```python
from build123d import *

# Parameters (mm, degrees)
SKETCH1_R           = 30.5
SKETCH1_R_2         = 25
BOSS_EXTRUDE1_DEPTH = 1
SKETCH2_R           = 30.5
SKETCH2_R_2         = 29.5
BOSS_EXTRUDE2_DEPTH = 10
SKETCH3_R           = 30.5
SKETCH3_R_2         = 25
BOSS_EXTRUDE3_DEPTH = 1


with BuildPart() as part:
    # Sketch1 → Boss-Extrude1 (new body)
    with BuildSketch(Plane.XY):
        Circle(SKETCH1_R)
        Circle(SKETCH1_R_2, mode=Mode.SUBTRACT)
    extrude(amount=BOSS_EXTRUDE1_DEPTH)

    # Sketch2 → Boss-Extrude2 (add)
    with BuildSketch(Plane(origin=(0, 0, 0), x_dir=(-1, 0, 0), z_dir=(0, 0, -1))):
        Circle(SKETCH2_R)
        Circle(SKETCH2_R_2, mode=Mode.SUBTRACT)
    extrude(amount=BOSS_EXTRUDE2_DEPTH)

    # Sketch3 → Boss-Extrude3 (add)
    with BuildSketch(Plane(origin=(0, 0, -10), x_dir=(-1, 0, 0), z_dir=(0, 0, -1))):
        Circle(SKETCH3_R)
        Circle(SKETCH3_R_2, mode=Mode.SUBTRACT)
    extrude(amount=BOSS_EXTRUDE3_DEPTH)


solid = part.part
```
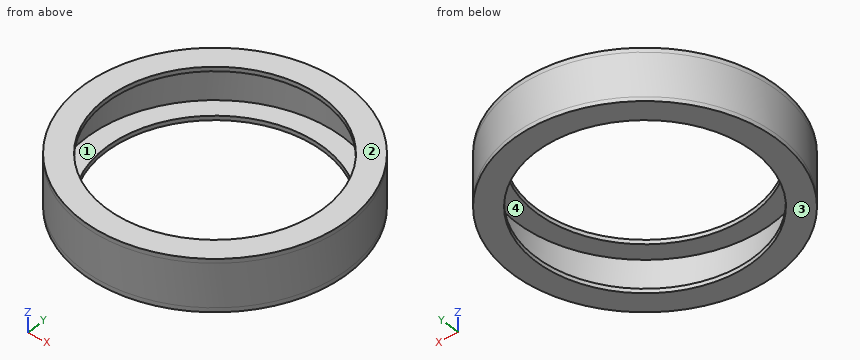
CAD build for the part. Positions are in the model's coordinates, mm. Face numbers are marked on the shaded views. A direction names the side the tool comes from. Coordinates: 2 decimals unless noted, no trailing zeros. Order: outer loops, then holes, each group sorted by start corner. A loop starts at its lowest first (then second) coordinate and runs counter-clockwise, first axis right, second up. Notation, with made-up numbers: M -2,76.25 L 55,76.25 A16 ccw 55,81.25 Z; hole C -9,38.5 d5. An arc over 180 degrees is marked long. Answer as CSV lines item,"result".
1) Mould opens along Y. For the marked faces 1 and 2 say: released by +Y, released by -Y, zero draft, split by the parting line, or undercut.
Verdict:
face 1,"undercut"
face 2,"zero draft"
2) 3-axis set-ups, long thin cutter, end or side, ignore diameter. For the marked faces 3 and 4: which of +Z, -Z, +X, -X, +Y, -Y reach the whole face in a straight line?
Verdict:
face 3,"-Z, +X, -X, +Y, -Y"
face 4,"none"
3) Flat gauge pins, fed straight in: P1, Ø2, axis at x = 17, z = -4, coming from the +Y side; P2, Ø2, axis at y = 11, z = -3.5, coming from the -X side; P3, Ø2, axis at y = 8.5, z = -10, coming from the -X side; P4, Ø4, axis at y = 1.5, z = -7.5, coming from the -X side. Where does each tip first touch, or does it go through?
Verdict:
P1,"y = 25.97"
P2,"x = -28.81"
P3,"x = -29.56"
P4,"x = -30.5"
4) Drill centre lines: L1, parallel to Z at x = -9, y = -23.5; L2, parallel to Y at x = 0, z = 0.55; L3, parallel to Y at x = 0.5, z = -5.75. Where is each one in solid material? Low to high. Write a range as from..to.
Verdict:
L1,"-11..-10, 0..1"
L2,"-30.5..-25, 25..30.5"
L3,"-30.5..-29.5, 29.5..30.5"
5) Cut at A-A (y = 0). List the corners of the cut face in (x, z).
Verdict:
outline,"M -30.5,-11 L -25,-11 L -25,-10 L -29.5,-10 L -29.5,0 L -25,0 L -25,1 L -30.5,1 Z; M 25,-11 L 30.5,-11 L 30.5,1 L 25,1 L 25,0 L 29.5,0 L 29.5,-10 L 25,-10 Z"
6) Cut at C-C (z = -5). List the corners of the cut face in (x, y).
Verdict:
outline,"C 0,0 d61; hole C 0,0 d59"
